Here's how the part is built. I have some questions about the finished solid (model axes, mm). A direction names the side the tool comes from. Round coordinates to 2 decimals unless told otherwise and drop trailing zeros. Write each loop counter-clockwise with the first axis right and the second up, starting at its lowest first coordinate (ties: lowest second). Pieces come first, ordered by that corner, then holes. Notation, with made-up numbers: (-38.5, -1) - (12.5, -1) arc R26 cw to (12.5, 15) - close; hole circle Ø3 at (51.5, 88). An arc over 180 degrees is marked (long way). Write item = value, one per line. Start each with the question number.
Item 1: For P1, Ø1.8, axis at y = 21.5, z = 7, coming from the +X side; P2, Ø6.5, axis at y = -23.5, z = 7.5, coming from the -X side; P3, Ø12, axis at x = 28, z = 20.5, coming from the -Y side, each with a flat end and sliding along its axis, tell me the tip position at first contact or that it passes through.
Item 2: If I drill on line 1 along Y through (x, z) = (-17.5, 8); line 2 along Z through (x, y) = (9, 0.5); line 3 along Z through (x, y) = (34.5, 9), over which ranges is the centre line in solid material (lowest first)? Write a range as [from, to].
Item 3: Which directions (+Z, -Z, +X, -X, +Y, -Y) give clear straight access to the entire face, cutting with the end or side of a thin tool? Please do faces 1 (the face through (12.5, 15, 2)), 2 (the face through (-44, 19, 6)), 3 (the face through (1, 5, 12)), 4 (the face through (44, 19, 6)).
Item 4: If we section it at A-A (x = -32): Please give me the cut outline in (y, z), and give its area (3 significant figures).
Item 5: Thinking about a two-plate mould opening in X: for faces 5 (the face through (-38, -22, 6)), 6 (the face through (31, 15, 0)), 7 (the face through (7.5, 0, 54)), which applies, pulls with the +X half, pulls with the -X half, needs draft (parallel to the pull), parting line crosses it, or undercut?
```python
from build123d import *

# Parameters (mm, degrees)
SKETCH002_W     = 30
SKETCH002_H     = 15
SKETCH001_W     = 60
SKETCH001_H     = 40
PAD_DEPTH       = 12
SKETCH003_W     = 10
SKETCH003_H     = 25
POCKET_DEPTH    = 100.001
SKETCH004_W     = 15
SKETCH004_H     = 31.516928
POCKET001_DEPTH = 20
SKETCH005_W     = 25
SKETCH005_H     = 5
POCKET002_DEPTH = 50.001


with BuildPart() as loft_body:
    # Sketch002 → Loft section 0
    with BuildSketch(Plane.XY.offset(64)):
        Rectangle(SKETCH002_W, SKETCH002_H)
    # Sketch001 → Loft section 1
    with BuildSketch(Plane.XY.offset(12)):
        with Locations((0.31551, 0)):
            Rectangle(SKETCH001_W, SKETCH001_H)
    loft()


with BuildPart() as pocket002:
    # Sketch → Pad (new body)
    with BuildSketch(Plane.XY):
        Polygon((-38, -25), (38, -25), (38, -19), (50, -19), (50, 19), (38, 19), (38, 25), (-38, 25), (-38, 19), (-50, 19), (-50, -19), (-38, -19), align=None)
    extrude(amount=PAD_DEPTH)

    # Fusion: union Loft body
    add(loft_body.part)

    # Sketch003 → Pocket (cut, through all)
    with BuildSketch(Plane.YZ.offset(50)):
        with Locations((0, 12.5)):
            Rectangle(SKETCH003_W, SKETCH003_H)
    extrude(amount=-POCKET_DEPTH, mode=Mode.SUBTRACT)

    # Sketch004 → Pocket001 (cut)
    with BuildSketch(Plane.XY.offset(64)):
        Rectangle(SKETCH004_W, SKETCH004_H)
    extrude(amount=-POCKET001_DEPTH, mode=Mode.SUBTRACT)

    # Sketch005 → Pocket002 (cut, through all)
    with BuildSketch(Plane.XZ.offset(25)):
        with Locations((0, 2.5)):
            Rectangle(SKETCH005_W, SKETCH005_H)
    extrude(amount=-POCKET002_DEPTH, mode=Mode.SUBTRACT)


solid = pocket002.part
```
Reply:
q1.P1 = 38
q1.P2 = -38
q1.P3 = -19.4
q2.line_1 = [-25, -5], [5, 25]
q2.line_2 = [25, 64]
q2.line_3 = [0, 12]
q3.face_1 = -Z, +Y, -Y
q3.face_2 = +Z, -Z, -X, +Y
q3.face_3 = -Z, +X, -X
q3.face_4 = +Z, -Z, +X, +Y
q4.outline = (-25, 0) - (-5, 0) - (-5, 12) - (-25, 12) - close; (5, 0) - (25, 0) - (25, 12) - (5, 12) - close
q4.area = 480 mm2
q5.face_5 = pulls with the -X half
q5.face_6 = needs draft
q5.face_7 = undercut
